from build123d import *

# Parameters (mm, degrees)
BOSS_EXTRUDE1_DEPTH      = 1.5875
BOSS_EXTRUDE1_DEPTH_BACK = 1.5875
SKETCH1_W                = 255.27
SKETCH1_H                = 73.96988
SKETCH1_R                = 1.5
SKETCH1_R_2              = 2.38125
BOSS_EXTRUDE2_DEPTH      = 3.175
BOSS_EXTRUDE2_DEPTH_BACK = 3.175
SKETCH1_4_W              = 255.27
SKETCH1_4_H              = 73.96988
CUT_EXTRUDE1_DEPTH       = 1.5875
CUT_EXTRUDE2_DEPTH       = 3.175
CUT_EXTRUDE2_DEPTH_BACK  = 3.175
SKETCH1_6_R              = 1.5


with BuildPart() as part:
    # Sketch1 → Boss-Extrude1 (new, two sides: drawn at the far end of the back side and taken through both)
    # profile 1 of 3: a face of its own
    with BuildSketch(Plane(origin=(0, 0, 0), x_dir=(1, 0, 0), z_dir=(0, 1, 0)).offset(-BOSS_EXTRUDE1_DEPTH_BACK)):
        with Locations((127.635, 36.98494)):
            Rectangle(SKETCH1_W, SKETCH1_H)
        with Locations(Location((178.435, 68.57238, 0), (0, 0, 270))):
            Circle(SKETCH1_R, mode=Mode.SUBTRACT)
        with Locations(Location((178.435, 5.3975, 0), (0, 0, 270))):
            Circle(SKETCH1_R, mode=Mode.SUBTRACT)
        with Locations(Location((229.235, 68.57238, 0), (0, 0, 270))):
            Circle(SKETCH1_R, mode=Mode.SUBTRACT)
        with Locations(Location((229.235, 5.3975, 0), (0, 0, 270))):
            Circle(SKETCH1_R, mode=Mode.SUBTRACT)
        with Locations(Location((127.635, 68.57238, 0), (0, 0, 270))):
            Circle(SKETCH1_R, mode=Mode.SUBTRACT)
        with Locations(Location((127.635, 5.3975, 0), (0, 0, 270))):
            Circle(SKETCH1_R, mode=Mode.SUBTRACT)
        with Locations(Location((26.035, 5.3975, 0), (0, 0, 270))):
            Circle(SKETCH1_R, mode=Mode.SUBTRACT)
        with Locations(Location((76.835, 5.3975, 0), (0, 0, 270))):
            Circle(SKETCH1_R, mode=Mode.SUBTRACT)
        with Locations(Location((26.035, 68.57238, 0), (0, 0, 270))):
            Circle(SKETCH1_R, mode=Mode.SUBTRACT)
        with Locations(Location((76.835, 68.57238, 0), (0, 0, 270))):
            Circle(SKETCH1_R, mode=Mode.SUBTRACT)
    # profile 2 of 3: a face of its own
    with BuildSketch(Plane(origin=(0, 0, 0), x_dir=(1, 0, 0), z_dir=(0, 1, 0)).offset(-BOSS_EXTRUDE1_DEPTH_BACK)):
        with BuildLine():
            Line((0, 62.38494), (-12.7, 62.38494))
            ThreePointArc((-12.7, 62.38494), (-17.190128061, 60.525068061), (-19.05, 56.03494))
            Line((-19.05, 56.03494), (-19.05, 17.93494))
            ThreePointArc((-19.05, 17.93494), (-17.190128061, 13.444811939), (-12.7, 11.58494))
            Line((-12.7, 11.58494), (0, 11.58494))
            Line((0, 11.58494), (0, 62.38494))
        make_face()
        with Locations(Location((-12.7, 56.03494, 0), (0, 0, 270))):
            Circle(SKETCH1_R_2, mode=Mode.SUBTRACT)
        with Locations(Location((-12.7, 17.93494, 0), (0, 0, 270))):
            Circle(SKETCH1_R_2, mode=Mode.SUBTRACT)
        with Locations(Location((-12.7, 36.98494, 0), (0, 0, 270))):
            Circle(SKETCH1_R_2, mode=Mode.SUBTRACT)
    # profile 3 of 3: a face of its own
    with BuildSketch(Plane(origin=(0, 0, 0), x_dir=(1, 0, 0), z_dir=(0, 1, 0)).offset(-BOSS_EXTRUDE1_DEPTH_BACK)):
        with BuildLine():
            Line((274.32, 56.03494), (274.32, 17.93494))
            ThreePointArc((274.32, 17.93494), (272.460128061, 13.444811939), (267.97, 11.58494))
            Line((267.97, 11.58494), (255.27, 11.58494))
            Line((255.27, 11.58494), (255.27, 62.38494))
            Line((255.27, 62.38494), (267.97, 62.38494))
            ThreePointArc((267.97, 62.38494), (272.460128061, 60.525068061), (274.32, 56.03494))
        make_face()
        with Locations(Location((267.97, 17.93494, 0), (0, 0, 270))):
            Circle(SKETCH1_R_2, mode=Mode.SUBTRACT)
        with Locations(Location((267.97, 56.03494, 0), (0, 0, 270))):
            Circle(SKETCH1_R_2, mode=Mode.SUBTRACT)
        with Locations(Location((267.97, 36.98494, 0), (0, 0, 270))):
            Circle(SKETCH1_R_2, mode=Mode.SUBTRACT)
    extrude(amount=BOSS_EXTRUDE1_DEPTH + BOSS_EXTRUDE1_DEPTH_BACK)

    # Sketch1_4 → Boss-Extrude2 (add, two sides: drawn at the far end of the back side and taken through both)
    with BuildSketch(Plane(origin=(0, 0, 0), x_dir=(1, 0, 0), z_dir=(0, 1, 0)).offset(-BOSS_EXTRUDE2_DEPTH_BACK)):
        with Locations((127.635, 36.98494)):
            Rectangle(SKETCH1_4_W, SKETCH1_4_H)
    extrude(amount=BOSS_EXTRUDE2_DEPTH + BOSS_EXTRUDE2_DEPTH_BACK)

    # Sketch2 → Cut-Extrude1 (cut)
    with BuildSketch(Plane(origin=(0, 3.175, 0), x_dir=(1, 0, 0), z_dir=(0, 1, 0))):
        with BuildLine():
            Line((13.335, 63.80988), (241.935, 63.80988))
            ThreePointArc((241.935, 63.80988), (244.18006403, 62.87994403), (245.11, 60.63488))
            Line((245.11, 60.63488), (245.11, 13.335))
            ThreePointArc((245.11, 13.335), (244.18006403, 11.08993597), (241.935, 10.16))
            Line((241.935, 10.16), (13.335, 10.16))
            ThreePointArc((13.335, 10.16), (11.08993597, 11.08993597), (10.16, 13.335))
            Line((10.16, 13.335), (10.16, 60.63488))
            ThreePointArc((10.16, 60.63488), (11.08993597, 62.87994403), (13.335, 63.80988))
        make_face()
    cut_extrude1 = extrude(amount=-CUT_EXTRUDE1_DEPTH, mode=Mode.SUBTRACT)

    # Mirror1: Cut-Extrude1 across plane
    add(cut_extrude1.mirror(Plane.ZX), mode=Mode.SUBTRACT)

    # Sketch1_6 → Cut-Extrude2 (cut, two sides: drawn at the far end of the back side and taken through both)
    with BuildSketch(Plane(origin=(0, 0, 0), x_dir=(1, 0, 0), z_dir=(0, 1, 0)).offset(-CUT_EXTRUDE2_DEPTH_BACK)):
        with Locations(Location((178.435, 68.57238, 0), (0, 0, 270))):
            Circle(SKETCH1_6_R)
        with Locations(Location((178.435, 5.3975, 0), (0, 0, 90))):
            Circle(SKETCH1_6_R)
        with Locations(Location((229.235, 68.57238, 0), (0, 0, 270))):
            Circle(SKETCH1_6_R)
        with Locations(Location((229.235, 5.3975, 0), (0, 0, 90))):
            Circle(SKETCH1_6_R)
        with Locations(Location((127.635, 68.57238, 0), (0, 0, 270))):
            Circle(SKETCH1_6_R)
        with Locations(Location((127.635, 5.3975, 0), (0, 0, 90))):
            Circle(SKETCH1_6_R)
        with Locations(Location((26.035, 5.3975, 0), (0, 0, 270))):
            Circle(SKETCH1_6_R)
        with Locations(Location((76.835, 5.3975, 0), (0, 0, 270))):
            Circle(SKETCH1_6_R)
        with Locations(Location((26.035, 68.57238, 0), (0, 0, 90))):
            Circle(SKETCH1_6_R)
        with Locations(Location((76.835, 68.57238, 0), (0, 0, 90))):
            Circle(SKETCH1_6_R)
    extrude(amount=CUT_EXTRUDE2_DEPTH + CUT_EXTRUDE2_DEPTH_BACK, mode=Mode.SUBTRACT)


solid = part.part
Can you work these out from the model? Positions are in its coordinate system, mm. A direction names the side the tool comes from. Coordinates: 2 decimals unless noted, no trailing zeros. Loops run counter-clockwise (first coordinate to the right, second up) from the corner with the lowest first, then second, coordinate; pieces in that order, holes last. Notation, with made-up numbers: (78, 65) - (131, 65) arc R13 cw to (131, 73) - close; hole circle Ø10 at (-3.75, 37.5). An arc over 180 degrees is marked (long way). Answer as a JSON object with one key per item and string values. Group by question number.
Item 1: If I drill on L1, parallel to Z at x = 267.97, y = -0.75; L2, parallel to X at y = 0.5, z = -17.5; L3, parallel to X at y = -2, z = -30.5, over which ranges is the centre line in solid material (lowest first)? Write a range as from..to.
Item 2: If we section it at A-A (x = 93.5): List the corners of the cut face in (y, z) for me (1 decimal), plus the area to 3 significant figures.
Item 3: If we mould it in two halves opening along X, with no side actions, what happens to faces 5 (the face through (255.27, -2, -36)), 6 (the face through (-11.1, 0, -57.8)), 7 (the face through (-11.1, 0, -19.7)), 8 (the face through (0, -2, -36))? For each: released by +X, released by -X, zero draft, split by the parting line, or undercut.
Item 4: On a 3-axis mill with a long thin cutter (end or side, diameter ignored), from which of +Z, -Z, +X, -X, +Y, -Y can I reach the whole of each face in a straight line? I mean faces 1 (the face through (129, 1.588, -37)), 2 (the face through (272.509, -0.022, -13.494)), 3 (the face through (129, -1.588, -37)), 4 (the face through (-10, -1.588, -37)). Say none if no direction works.
Item 5: For pin 1 (1.3 mm diameter, centred on y = -2, z = -37.5, fed in from +X); pin 2 (1.3 mm diameter, centred on y = -2.5, z = -37, fed in from -X); pin 3 (0.5 mm diameter, centred on y = 2, z = -40.5, fed in from +X); pin 4 (6 mm diameter, centred on x = 74, z = -33.5, fed in from -Y), each with a flat end and sliding along its axis, tell me the tip position at first contact or that it passes through.
Returned:
{
 "1": {"L1": "z = -62.38..-58.42, -53.65..-39.37, -34.6..-20.32, -15.55..-11.58", "L2": "x = -19.04..-15.04, -10.36..265.63, 270.31..274.31", "L3": "x = 0..10.16, 245.11..255.27"},
 "2": {"outline": "(-3.2, -74) - (3.2, -74) - (3.2, -63.8) - (1.6, -63.8) - (1.6, -10.2) - (3.2, -10.2) - (3.2, 0) - (-3.2, 0) - (-3.2, -10.2) - (-1.6, -10.2) - (-1.6, -63.8) - (-3.2, -63.8) - close", "area": "299 mm²"},
 "3": {"face 5": "released by +X", "face 6": "undercut", "face 7": "undercut", "face 8": "released by -X"},
 "4": {"face 1": "+Y", "face 2": "+Z, +X, +Y, -Y", "face 3": "-Y", "face 4": "+Z, -Z, -X, -Y"},
 "5": {"pin 1": "stops at x = 274.32", "pin 2": "stops at x = 0", "pin 3": "stops at x = 255.27", "pin 4": "stops at y = -1.59"}
}
